```python
from build123d import *

# Parameters (mm, degrees)
BOSS_EXTRUDE1_DEPTH = 2


with BuildPart() as part:
    # Sketch1 → Boss-Extrude1 (new body)
    with BuildSketch(Plane(origin=(0, 0, 0), x_dir=(1, 0, 0), z_dir=(0, 1, 0))):
        with BuildLine():
            Line((25, 55), (21.109165494, 42.59796501))
            Line((21.109165494, 42.59796501), (26.118434554, 41.026429618))
            Line((26.118434554, 41.026429618), (30.502299771, 55))
            Line((30.502299771, 55), (216.654895807, 55))
            Line((216.654895807, 55), (221.038761024, 41.026429618))
            Line((221.038761024, 41.026429618), (226.048030084, 42.59796501))
            Line((226.048030084, 42.59796501), (222.157195577, 55))
            Line((222.157195577, 55), (242.157195577, 55))
            ThreePointArc((242.157195577, 55), (245.692729483, 53.535533906), (247.157195577, 50))
            Line((247.157195577, 50), (247.157195577, 5))
            ThreePointArc((247.157195577, 5), (245.692729483, 1.464466094), (242.157195577, 0))
            Line((242.157195577, 0), (239.412097536, 0))
            Line((239.412097536, 0), (235.028232319, 13.973570382))
            Line((235.028232319, 13.973570382), (230.018963259, 12.40203499))
            Line((230.018963259, 12.40203499), (233.909797765, 0))
            Line((233.909797765, 0), (13.247397812, 0))
            Line((13.247397812, 0), (17.138232319, 12.40203499))
            Line((17.138232319, 12.40203499), (12.128963259, 13.973570382))
            Line((12.128963259, 13.973570382), (7.745098042, 0))
            Line((7.745098042, 0), (5, 0))
            ThreePointArc((5, 0), (1.464466094, 1.464466094), (0, 5))
            Line((0, 5), (0, 50))
            ThreePointArc((0, 50), (1.464466094, 53.535533906), (5, 55))
            Line((5, 55), (25, 55))
        make_face()
    extrude(amount=BOSS_EXTRUDE1_DEPTH)


solid = part.part
```
Here's how the part is built. I have some questions about the finished solid (model axes, mm). A direction names the side the tool comes from. Round coordinates to 2 decimals unless told otherwise and drop trailing zeros. Order: outer loops, then holes, each group sorted by start corner. A loop starts at its lowest first (then second) coordinate and runs counter-clockwise, first axis right, second up. Notation, with made-up numbers: M 80.25,39 L 87.25,39 A28 ccw 87.25,72 Z; hole C 86.25,-25 d3. An arc over 180 degrees is marked long. Answer in a Markdown table with one row per item.
Item 1: Imagine slicing it at A-A, the plane y = 1.6. Write out the boundary of the cut face in (x, z), and give its area (3 significant figures).
A:
| item | result |
|---|---|
| outline | M 0,-50 A5 ccw 5,-55 L 25,-55 L 21.11,-42.6 L 26.12,-41.03 L 30.5,-55 L 216.65,-55 L 221.04,-41.03 L 226.05,-42.6 L 222.16,-55 L 242.16,-55 A5 ccw 247.16,-50 L 247.16,-5 A5 ccw 242.16,0 L 239.41,0 L 235.03,-13.97 L 230.02,-12.4 L 233.91,0 L 13.25,0 L 17.14,-12.4 L 12.13,-13.97 L 7.75,0 L 5,0 A5 ccw 0,-5 Z |
| area | 13,300 mm2 |
Item 2: For faces 4 (the face through (231.937, 0.986, -6.288)), 5 (the face through (9.968, 0.986, -7.085)), 6 (the face through (218.816, 0.986, -48.111)), 7 (the face through (125, 0, -28)), 8 (the face through (1, 1, -53)), which set-ups out of +Z, -Z, +X, -X, +Y, -Y let a thin tool reach every point of the face, with its end or its side?
A:
| item | result |
|---|---|
| face 4 | +Y, -Y |
| face 5 | +Z, +Y, -Y |
| face 6 | -Z, +Y, -Y |
| face 7 | +Z, -Z, +X, -X, -Y |
| face 8 | -Z, -X, +Y, -Y |
Item 3: Thinking about a two-plate mould opening in Z: for faces 1 (the face through (28.28, 0.99, -47.92)), 2 (the face through (237.25, 0.99, -6.89)), 3 (the face through (224.13, 0.99, -48.71)), which applies, +Z half, -Z half, draft (parallel to the pull), parting line (faces both ways), or undercut?
A:
| item | result |
|---|---|
| face 1 | -Z half |
| face 2 | +Z half |
| face 3 | undercut |
Item 4: If I drill on L1, parallel to X at y = 1.8, z = -5.5; L2, parallel to X at y = 0.55, z = -49.5, over which ranges is the centre line in solid material (lowest first)? Write a range as from..to.
A:
| item | result |
|---|---|
| L1 | x = 0..9.47, 14.97..232.18, 237.69..247.16 |
| L2 | x = 0..23.27, 28.78..218.38, 223.88..247.16 |
